Verification items for the finished model (mm, model axes). Face numbers are marked on the shaded views. A direction names the side the tool comes from. Round coordinates to 2 decimals unless told otherwise and drop trailing zeros. Write each loop counter-clockwise with the first axis right and the second up, starting at its lowest first coordinate (ties: lowest second). Pieces come first, ordered by that corner, then holes. Notation, with made-up numbers: M -20,21.5 L -5,21.5 A22 cw -5,34.5 Z; hole C -1.75,41 d10. An arc over 180 degrees is marked long. Answer in a Markdown table with one row per item. Add a question column.
1. Set-up check for the marked faces 5 and 6: record each of +Z, -Z, +X, -X, +Y, -Y from which the full face is reachable in a straight line by a thin tool's end or side.
2. Sectioned sample at C-C on z = -9.5. Record the cut outline in (x, y).
3. Sectioned sample at B-B on x = 0. Record the cut outline in (y, z), plus the area to 3 significant figures.
4. Draft check along Z on the marked faces 1, 2, 3 and 4. Enter one of: pulls with the +Z half, pulls with the -Z half, needs draft (parallel to the pull), parting line crosses it, or undercut.
5. Go/stop test with flat-tipped pins: pin 1 Ø3 at (x, z) = (-11, 10) entering from +Y; pin 2 Ø1.8 at (x, z) = (-10.25, -3.75) entering from +Y; pin 3 Ø1.5 at (x, y) = (6, 3) entering from -Z; pin 4 Ø9.5 at (x, z) = (0, 3.91) entering from -Y. Record where each tip stops, or that it passes through.
6. Sectioned sample at A-A on y = 5. Count the separate pieces of the cut face and the enclosed holes in it, plus the area to 3 significant figures.
7. Material ranges on probe 1 along Z at (x, y) = (-10.25, 7); probe 2 along X at (y, z) = (11, 0.5); probe 3 along X at (y, z) = (8, 9.75), recorded low to high.
8. Sectioned sample at D-D on x = -6.5. Record the cut outline in (y, z), plus the area to 3 significant figures.
```python
from build123d import *

# Parameters (mm, degrees)
CROQUIS1_W                 = 30
CROQUIS1_H                 = 29
SALIENTE_EXTRUIR1_DEPTH    = 15.5
CROQUIS2_W                 = 25.5
CROQUIS2_H                 = 24.5
CORTAR_EXTRUIR1_DEPTH      = 14.5
REDONDEO1_R                = 2
CROQUIS5_R                 = 6
CORTAR_EXTRUIR3_DEPTH      = 5
CORTAR_EXTRUIR5_DEPTH      = 0.75
CORTAR_EXTRUIR5_DEPTH_BACK = 3
CROQUIS6_W                 = 25.5
CROQUIS6_H                 = 13.5
CROQUIS3_R                 = 1.75
CROQUIS3_R_2               = 1
SALIENTE_EXTRUIR2_DEPTH    = 9.5


with BuildPart() as part:
    # Croquis1 → Saliente-Extruir1 (new body)
    with BuildSketch(Plane(origin=(0, 0, 0), x_dir=(1, 0, 0), z_dir=(0, 1, 0))):
        Rectangle(CROQUIS1_W, CROQUIS1_H)
    extrude(amount=SALIENTE_EXTRUIR1_DEPTH)

    # Croquis2 → Cortar-Extruir1 (cut)
    with BuildSketch(Plane(origin=(0, 15.5, 0), x_dir=(1, 0, 0), z_dir=(0, 1, 0))):
        Rectangle(CROQUIS2_W, CROQUIS2_H)
    extrude(amount=-CORTAR_EXTRUIR1_DEPTH, mode=Mode.SUBTRACT)

    # Redondeo1
    redondeo1_edges = [part.edges().sort_by_distance(p)[0] for p in [
        (0, 0, -14.5),
        (15, 0, 0),
        (0, 0, 14.5),
        (-15, 0, 0),
    ]]
    fillet(redondeo1_edges, radius=REDONDEO1_R)

    # Croquis5 → Cortar-Extruir3 (cut)
    with BuildSketch(Plane(origin=(0, 1, 0), x_dir=(1, 0, 0), z_dir=(0, 1, 0))):
        with Locations(Location((0, -3.907682746, 0), (0, 0, 270))):
            Circle(CROQUIS5_R)
    extrude(amount=-CORTAR_EXTRUIR3_DEPTH, mode=Mode.SUBTRACT)

    # Croquis6 → Cortar-Extruir5 (cut, two sides: drawn at the far end of the back side and taken through both)
    with BuildSketch(Plane(origin=(0, 0, -14.5), x_dir=(-1, 0, 0), z_dir=(0, 0, -1)).offset(-CORTAR_EXTRUIR5_DEPTH_BACK)):
        with Locations((0, 8.75)):
            Rectangle(CROQUIS6_W, CROQUIS6_H)
    extrude(amount=CORTAR_EXTRUIR5_DEPTH + CORTAR_EXTRUIR5_DEPTH_BACK, mode=Mode.SUBTRACT)

    # Croquis3 → Saliente-Extruir2 (add)
    # profile 1 of 4: a face of its own
    with BuildSketch(Plane(origin=(0, 1, 0), x_dir=(1, 0, 0), z_dir=(0, 1, 0))):
        with Locations(Location((10.25, -9.75, 0), (0, 0, 90))):
            Circle(CROQUIS3_R)
        with Locations(Location((10.25, -9.75, 0), (0, 0, 270))):
            Circle(CROQUIS3_R_2, mode=Mode.SUBTRACT)
    # profile 2 of 4: a face of its own
    with BuildSketch(Plane(origin=(0, 1, 0), x_dir=(1, 0, 0), z_dir=(0, 1, 0))):
        with Locations(Location((10.25, 3.75, 0), (0, 0, 90))):
            Circle(CROQUIS3_R)
        with Locations(Location((10.25, 3.75, 0), (0, 0, 270))):
            Circle(CROQUIS3_R_2, mode=Mode.SUBTRACT)
    # profile 3 of 4: a face of its own
    with BuildSketch(Plane(origin=(0, 1, 0), x_dir=(1, 0, 0), z_dir=(0, 1, 0))):
        with Locations(Location((-10.25, 3.75, 0), (0, 0, 90))):
            Circle(CROQUIS3_R)
        with Locations(Location((-10.25, 3.75, 0), (0, 0, 90))):
            Circle(CROQUIS3_R_2, mode=Mode.SUBTRACT)
    # profile 4 of 4: a face of its own
    with BuildSketch(Plane(origin=(0, 1, 0), x_dir=(1, 0, 0), z_dir=(0, 1, 0))):
        with Locations(Location((-10.25, -9.75, 0), (0, 0, 90))):
            Circle(CROQUIS3_R)
        with Locations(Location((-10.25, -9.75, 0), (0, 0, 90))):
            Circle(CROQUIS3_R_2, mode=Mode.SUBTRACT)
    extrude(amount=SALIENTE_EXTRUIR2_DEPTH)


solid = part.part
```
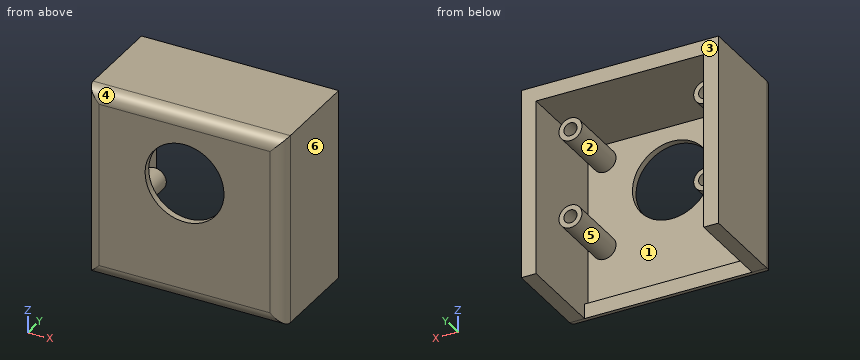
Geometry check:
| question | item | result |
|---|---|---|
| 1 | face 5 | +Y |
| 1 | face 6 | +Z, -Z, +X, +Y, -Y |
| 2 | outline | M -15,2 A2 ccw -13,0 L 13,0 A2 ccw 15,2 L 15,15.5 L 12.75,15.5 L 12.75,1 L -12.75,1 L -12.75,15.5 L -15,15.5 Z |
| 3 | outline | M 0,-12.5 A2 ccw 2,-14.5 L 2,-12.25 L 1,-12.25 L 1,-2.09 L 0,-2.09 Z; M 0,9.91 L 1,9.91 L 1,12.25 L 15.5,12.25 L 15.5,14.5 L 2,14.5 A2 ccw 0,12.5 Z |
| 3 | area | 50.2 mm2 |
| 4 | face 1 | undercut |
| 4 | face 2 | undercut |
| 4 | face 3 | needs draft |
| 4 | face 4 | pulls with the +Z half |
| 5 | pin 1 | stops at y = 10.5 |
| 5 | pin 2 | stops at y = 1 |
| 5 | pin 3 | stops at z = 12.25 |
| 5 | pin 4 | passes through |
| 6 | separate pieces | 5 |
| 6 | enclosed holes | 4 |
| 6 | area | 214 mm2 |
| 7 | probe 1 | z = -5.5 to -4.75, -2.75 to -2, 8 to 8.75, 10.75 to 11.5, 12.25 to 14.5 |
| 7 | probe 2 | x = -15 to -12.75, 12.75 to 15 |
| 7 | probe 3 | x = -15 to -12.75, -12 to -11.25, -9.25 to -8.5, 8.5 to 9.25, 11.25 to 12, 12.75 to 15 |
| 8 | outline | M 0,-12.5 A2 ccw 2,-14.5 L 2,-12.25 L 1,-12.25 L 1,12.25 L 15.5,12.25 L 15.5,14.5 L 2,14.5 A2 ccw 0,12.5 Z |
| 8 | area | 62.2 mm2 |
